The listing builds one solid part. Answer for the finished solid, in the listing's coordinates (mm). Face numbers are marked on the shaded views. Give positions to 0.01 mm unless a question says otherwise; leave off trailing zeros. Order: outer loops, then holes, each group sorted by start corner. A loop starts at its lowest first (then second) coordinate and runs counter-clockwise, first axis right, second up. Notation, with made-up numbers: (84.5, -30) - (109.5, -30) arc R6 ccw to (109.5, -26) - close; hole circle Ø10 at (37.25, -12). An arc over 180 degrees is marked (long way). Answer as a JSON object with one key per item and string values. Group by question number.
Q1. The mould has two halves that part along Y. Classify the marked faces 1, 2 and 3: released by +Y, released by -Y, zero draft, split by the parting line, or undercut.
Q2. A cutting plane is placed at B-B, the plane z = 13. Give the vertices of the cut face in (x, y), and give its area (3 significant figures).
Q3. A cutting plane is placed at A-A, the plane x = 0. Give the vertices of the cut face in (y, z), and give its area (3 significant figures).
Q4. Consider line 1 (X direction, y = 0.05, z = 23); line 2 (Z direction, x = -1.15, y = 1.05); line 3 (Y direction, x = -1.05, z = 10). Determine where each line is inside the solid, lowest interval first.
Q5. Given pin 1 (1.5 mm diameter, centred on x = 2, y = 2, fed in from -Z); pin 2 (1.5 mm diameter, centred on y = 0.5, z = 3, fed in from +X); pin 3 (1.5 mm diameter, centred on x = 0, y = -0.5, fed in from -Z); pin 4 (1 mm diameter, centred on x = 1, z = 26, fed in from -Y), each flat-ended and moving along its own axis, determine where each tip first touches the part or whether it passes through.
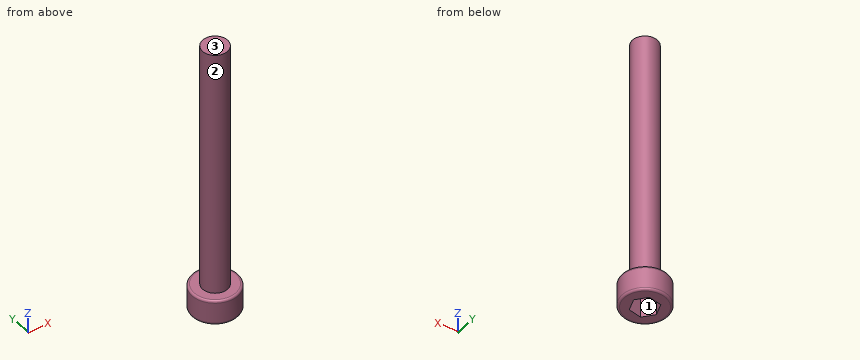
from build123d import *

# Parameters (mm, degrees)
SKETCH1_R           = 1.5
BOSS_EXTRUDE1_DEPTH = 30
SKETCH2_R           = 2.75
BOSS_EXTRUDE2_DEPTH = 3
FILLET1_R           = 0.254
CUT_EXTRUDE1_DEPTH  = 2.54


with BuildPart() as part:
    # Sketch1 → Boss-Extrude1 (new body)
    with BuildSketch(Plane.XY):
        Circle(SKETCH1_R)
    extrude(amount=BOSS_EXTRUDE1_DEPTH)

    # Sketch2 → Boss-Extrude2 (add)
    with BuildSketch(Plane(origin=(0, 0, 0), x_dir=(-1, 0, 0), z_dir=(0, 0, -1))):
        with Locations((0, 0.018427268)):
            Circle(SKETCH2_R)
    extrude(amount=BOSS_EXTRUDE2_DEPTH)

    # Fillet1
    fillet1_edges = [part.edges().sort_by_distance(p)[0] for p in [
        (2.75, 0.018427268, 0),
        (2.75, 0.018427268, -3),
    ]]
    fillet(fillet1_edges, radius=FILLET1_R)

    # Sketch3 → Cut-Extrude1 (cut)
    with BuildSketch(Plane(origin=(0, 0, -3), x_dir=(-1, 0, 0), z_dir=(0, 0, -1))):
        Polygon((1.570116236, -0.229317517), (0.999611396, 1.254315423), (-0.57050484, 1.502060208), (-1.570116236, 0.266172054), (-0.999611396, -1.217460886), (0.57050484, -1.465205671), align=None)
    extrude(amount=-CUT_EXTRUDE1_DEPTH, mode=Mode.SUBTRACT)


solid = part.part
Reply:
{
 "1": {"face 1": "undercut", "face 2": "split by the parting line", "face 3": "zero draft"},
 "2": {"outline": "circle Ø3 at (0, 0)", "area": "7.07 mm^2"},
 "3": {"outline": "(-2.73, -2.75) arc R0.25 ccw to (-2.48, -3) - (-1.38, -3) - (-1.38, -0.46) - (1.41, -0.46) - (1.41, -3) - (2.51, -3) arc R0.25 ccw to (2.77, -2.75) - (2.77, -0.25) arc R0.25 ccw to (2.51, 0) - (1.5, 0) - (1.5, 30) - (-1.5, 30) - (-1.5, 0) - (-2.48, 0) arc R0.25 ccw to (-2.73, -0.25) - close", "area": "99.4 mm^2"},
 "4": {"line 1": "x = -1.5 to 1.5", "line 2": "z = -3 to 0", "line 3": "y = -1.07 to 1.07"},
 "5": {"pin 1": "stops at z = -3", "pin 2": "stops at x = 1.5", "pin 3": "stops at z = -0.46", "pin 4": "stops at y = -1.41"}
}
